Build history of the part. All positions in model axes, mm. Face numbers are marked on the shaded views. A direction names the side the tool comes from. Give positions to 0.01 mm unless a question says otherwise; leave off trailing zeros. Write each loop counter-clockwise with the first axis right and the second up, starting at its lowest first coordinate (ties: lowest second). Pieces come first, ordered by that corner, then holes.
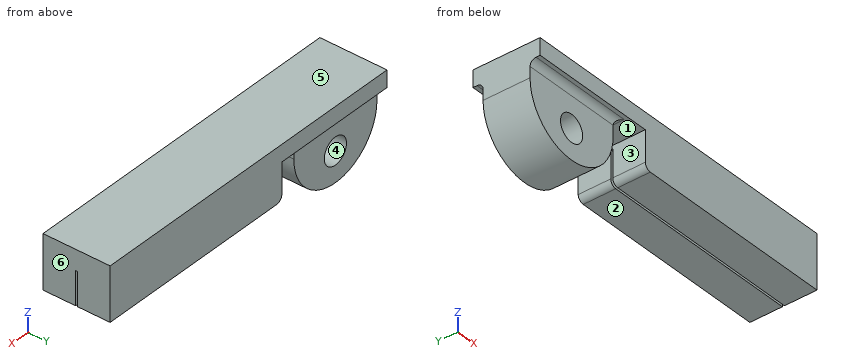
from build123d import *

# Parameters (mm, degrees)
F1_DEPTH = 10
F0_R     = 4
F2_DEPTH = 7
F3_R     = 1.8
F6_DEPTH = 65


with BuildPart() as f1:
    # F0 (on Front) → F1 (new body, symmetric)
    with BuildSketch(Plane.XZ):
        Polygon((100, 25), (0, 25), (0, 20), (30, 20), (38, 20), (38, 9), (100, 9), align=None)
    extrude(amount=F1_DEPTH, both=True)

    # F0 (on Front) → F2 (join, symmetric)
    with BuildSketch(Plane.XZ):
        Polygon((100, 25), (0, 25), (0, 20), (30, 20), (38, 20), (38, 9), (100, 9), align=None)
        with BuildLine():
            Line((30, 20), (0, 20))
            Line((0, 20), (0, 15))
            ThreePointArc((0, 15), (15, 0), (30, 15))
            Line((30, 15), (30, 20))
        make_face()
        with Locations((15, 9)):
            Circle(F0_R, mode=Mode.SUBTRACT)
    extrude(amount=F2_DEPTH, both=True)

    # F3
    f3_edges = [f1.edges().sort_by_distance(p)[0] for p in [
        (30, 0, 20),
        (15, -7, 20),
        (15, 7, 20),
        (38, 0, 9),
    ]]
    fillet(f3_edges, radius=F3_R)

    # F5 (on offset) → F6 (cut)
    with BuildSketch(Plane.YZ.offset(100)):
        Polygon((-0.3, 9), (0, 9), (0.3, 9), (0.3, 19), (-0.3, 19), align=None)
    extrude(amount=-F6_DEPTH, mode=Mode.SUBTRACT)


solid = f1.part
1. Mould opens along X. For the marked faces 4, 5 and 6 say: pulls with the +X half, pulls with the -X half, needs draft (parallel to the pull), parting line crosses it, or undercut.
2. Saw through at B-B on y = 5.75. Give the cut face in (x, z), plus the area to 3 significant figures.
3. Drop flat-ended pins along their axis: pin 1 (14.5 mm diameter, centred on x = 12.5, z = 7, fed in from -Y); pin 2 (5 mm diameter, centred on x = 58.5, y = -5, fed in from -Z); pin 3 (1.5 mm diameter, centred on y = -7.5, z = 5.5, fed in from +X); pin 4 (3 mm diameter, centred on y = -2.5, z = 14.5, fed in from -X). Give the stop position or say it passes through.
4. Saw through at A-A on x = 15. Give the cut face in (y, z).
5. Saw through at C-C on x = 77. Give the cut face in (y, z).
6. Saw through at D-D on x = 25. Give the cut face in (y, z), plus the area to 3 significant figures.
7. Drill centre lines: line 1 along Z through (x, y) = (15, -0.25); line 2 along Y through (x, z) = (79, 17.25); line 3 along Z through (x, y) = (83, -1). Where is each one in solid material? Low to high.
8. 3-axis set-ups, long thin cutter, end or side, ignore diameter. For the marked faces 1, 2 and 3: which of +Z, -Z, +X, -X, +Y, -Y reach the whole face in a straight line?
Outcome:
1. face 4: undercut
1. face 5: needs draft
1. face 6: pulls with the +X half
2. outline: (0, 15) arc R15 ccw to (30, 15) - (30, 18.2) arc R1.8 cw to (31.8, 20) - (38, 20) - (38, 10.8) arc R1.8 ccw to (39.8, 9) - (100, 9) - (100, 25) - (0, 25) - close; hole circle Ø8 at (15, 9)
2. area: 1,640 mm2
3. pin 1: stops at y = -7
3. pin 2: stops at z = 9
3. pin 3: stops at x = 27.04
3. pin 4: stops at x = 0
4. outline: (-10, 20) - (-8.8, 20) arc R1.8 cw to (-7, 18.2) - (-7, 13) - (7, 13) - (7, 18.2) arc R1.8 cw to (8.8, 20) - (10, 20) - (10, 25) - (-10, 25) - close; (-7, 0) - (7, 0) - (7, 5) - (-7, 5) - close
5. outline: (-10, 9) - (-0.3, 9) - (-0.3, 19) - (0.3, 19) - (0.3, 9) - (10, 9) - (10, 25) - (-10, 25) - close
6. outline: (-10, 20) - (-8.8, 20) arc R1.8 cw to (-7, 18.2) - (-7, 3.82) - (7, 3.82) - (7, 18.2) arc R1.8 cw to (8.8, 20) - (10, 20) - (10, 25) - (-10, 25) - close
6. area: 328 mm2
7. line 1: z = 0 to 5, 13 to 25
7. line 2: y = -10 to -0.3, 0.3 to 10
7. line 3: z = 9 to 25
8. face 1: -Z
8. face 2: -Z, +X, +Y, -Y
8. face 3: -Z, +Y, -Y
